The figure shows three views and two pictorial views of one solid part (mm, origin at its lowest corner). Answer the questions. Coordinates: 2 decimals unless noted, no trailing zeros. Write each loop counter-clockwise with the first axis right and the second up, starting at its lowest first coordinate (ties: lowest second). Pieces come first, ordered by that corner, then holes. Notation, with made-up numbers: (-7, 20.5) -> (47, 20.5) arc R26 cw to (47, 38.5) -> close; hole circle Ø5 at (-3, -31). An arc over 180 degrees is marked (long way). Use CSV: the item, a comma, the result in double quotes. Start each with the question number.
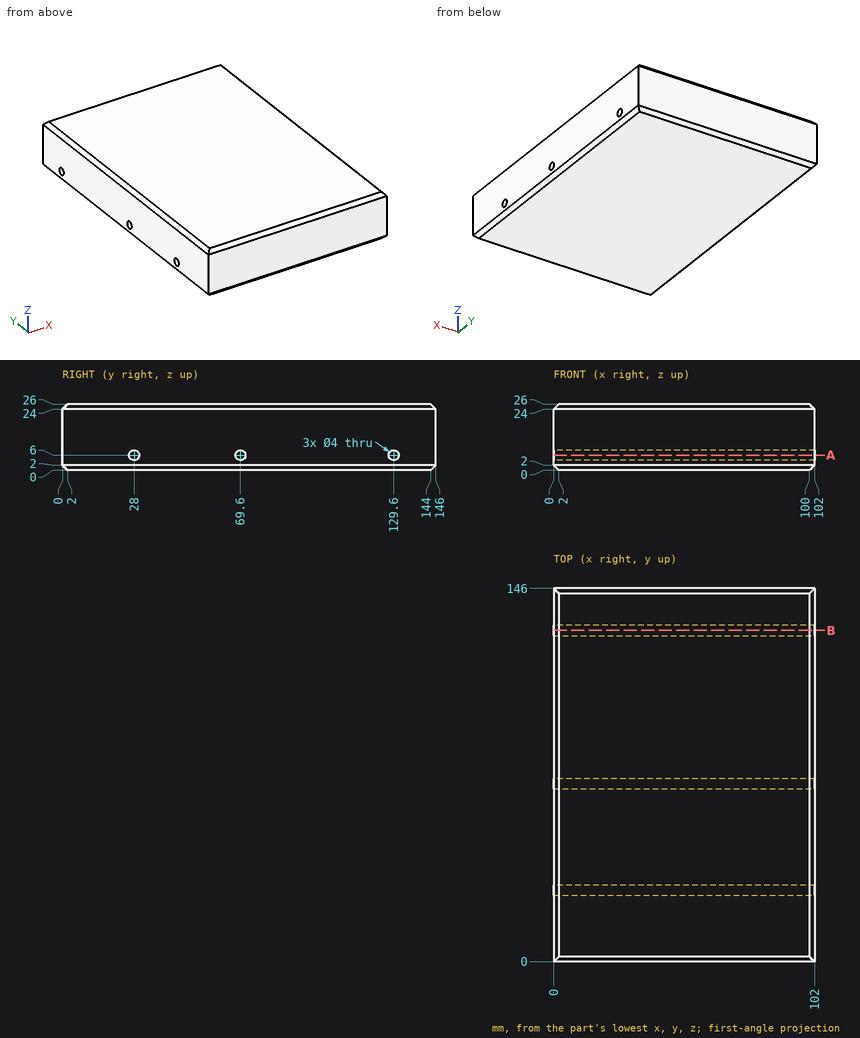
1) Section B-B, the plane y = 129.6 is taken. Give the vertices of the cut face in (x, z), plus the area to 3 significant figures.
2) Find the intervals of material crossed by line 1 along Z through (x, y) = (30, 129.6); line 2 along Y through (x, z) = (96, 5.25); line 3 along Y through (x, z) = (51, 7.25), in increasing order.
3) Section A-A, the plane z = 6 is taken. Give the vertices of the cut face in (x, y).
The answers:
1,outline,"(0, 2) -> (2, 0) -> (100, 0) -> (102, 2) -> (102, 4) -> (0, 4) -> close; (0, 8) -> (102, 8) -> (102, 24) -> (100, 26) -> (2, 26) -> (0, 24) -> close"
1,area,"2,240 mm^2"
2,line 1,"z = 0 to 4, 8 to 26"
2,line 2,"y = 0 to 26.15, 29.85 to 67.75, 71.45 to 127.75, 131.45 to 146"
2,line 3,"y = 0 to 26.44, 29.56 to 68.04, 71.16 to 128.04, 131.16 to 146"
3,outline,"(0, 0) -> (102, 0) -> (102, 26) -> (0, 26) -> close; (0, 30) -> (102, 30) -> (102, 67.6) -> (0, 67.6) -> close; (0, 71.6) -> (102, 71.6) -> (102, 127.6) -> (0, 127.6) -> close; (0, 131.6) -> (102, 131.6) -> (102, 146) -> (0, 146) -> close"
